```python
from build123d import *

# Parameters (mm, degrees)
SKETCH1_W           = 32.1
SKETCH1_H           = 32.1
SKETCH1_R           = 0.95
BOSS_EXTRUDE1_DEPTH = 1.65
SKETCH2_W           = 22.1
SKETCH2_H           = 6.75
BOSS_EXTRUDE2_DEPTH = 2.5
SKETCH3_R           = 0.625
BOSS_EXTRUDE3_DEPTH = 5
SKETCH4_R           = 7
BOSS_EXTRUDE4_DEPTH = 17


with BuildPart() as part:
    # Sketch1 → Boss-Extrude1 (new body)
    with BuildSketch(Plane(origin=(0, 0, 0), x_dir=(1, 0, 0), z_dir=(0, 1, 0))):
        Rectangle(SKETCH1_W, SKETCH1_H)
        with Locations(Location((-14.05, 14.05, 0), (0, 0, 270))):
            Circle(SKETCH1_R, mode=Mode.SUBTRACT)
        with Locations(Location((14.05, 14.05, 0), (0, 0, 90))):
            Circle(SKETCH1_R, mode=Mode.SUBTRACT)
        with Locations(Location((14.05, -14.05, 0), (0, 0, 270))):
            Circle(SKETCH1_R, mode=Mode.SUBTRACT)
        with Locations(Location((-14.05, -14.05, 0), (0, 0, 90))):
            Circle(SKETCH1_R, mode=Mode.SUBTRACT)
    extrude(amount=BOSS_EXTRUDE1_DEPTH)

    # Sketch2 → Boss-Extrude2 (add)
    with BuildSketch(Plane.XZ):
        with Locations((0, 12.675)):
            Rectangle(SKETCH2_W, SKETCH2_H)
    extrude(amount=BOSS_EXTRUDE2_DEPTH)

    # Sketch3 → Boss-Extrude3 (add)
    with BuildSketch(Plane(origin=(0, 1.65, 0), x_dir=(1, 0, 0), z_dir=(0, 1, 0))):
        with BuildLine():
            Line((9.9, 2.25), (8.55, 2.25))
            Line((8.55, 2.25), (8.55, 8.55))
            Line((8.55, 8.55), (-8.55, 8.55))
            Line((-8.55, 8.55), (-8.55, 2.25))
            Line((-8.55, 2.25), (-9.9, 2.25))
            ThreePointArc((-9.9, 2.25), (-12.15, 0), (-9.9, -2.25))
            Line((-9.9, -2.25), (-8.55, -2.25))
            Line((-8.55, -2.25), (-8.55, -8.55))
            Line((-8.55, -8.55), (8.55, -8.55))
            Line((8.55, -8.55), (8.55, -2.25))
            Line((8.55, -2.25), (9.9, -2.25))
            ThreePointArc((9.9, -2.25), (12.15, 0), (9.9, 2.25))
        make_face()
        with Locations(Location((9.9, 0, 0), (0, 0, 270))):
            Circle(SKETCH3_R, mode=Mode.SUBTRACT)
        with Locations(Location((-9.9, 0, 0), (0, 0, 90))):
            Circle(SKETCH3_R, mode=Mode.SUBTRACT)
    extrude(amount=BOSS_EXTRUDE3_DEPTH)

    # Sketch4 → Boss-Extrude4 (add)
    with BuildSketch(Plane(origin=(0, 6.65, 0), x_dir=(1, 0, 0), z_dir=(0, 1, 0))):
        with Locations(Location((0, 0, 0), (0, 0, 270))):
            Circle(SKETCH4_R)
    extrude(amount=BOSS_EXTRUDE4_DEPTH)


solid = part.part
```
The listing builds one solid part. Answer for the finished solid, in the listing's coordinates (mm). A direction names the side the tool comes from. Coordinates: 2 decimals unless noted, no trailing zeros. Write each loop counter-clockwise with the first axis right and the second up, starting at its lowest first coordinate (ties: lowest second). Pieces come first, ordered by that corner, then holes. Notation, with made-up numbers: M 7.25,9.5 L 61.25,9.5 A14 cw 61.25,20.5 Z; hole C -26,67.25 d7. An arc over 180 degrees is marked long. Use a Markdown table: item, result. Add a question column.
1. Section D-D (z = 10.5) is taken. Give the vertices of the cut face in (x, y).
2. Section C-C (x = 0) is taken. Give the vertices of the cut face in (y, z).
3. Which of the six approach directions +Z, -Z, +X, -X, +Y, -Y give full straight-line access (tool end or side, diameter ignored) to faces 1 (the flat face through (-9, 4, 2.25)), 2 (the flat face through (8.55, 4, -5)), 3 (the flat face through (10, 1.65, 0))?
4. Straight lines are drawn through the part: line 1 along X through (y, z) = (1.1, -14.05); line 2 along X through (y, z) = (3.85, 0) (3 decimals); line 3 along Y through (x, z) = (-12, -5.5). For each, find the intervals that lie inside material, in ascending order. Write a range as [from, to].
5. Given P1, Ø12, axis at x = 9.5, y = 20, coming from the +Z side; P2, Ø8, axis at x = -4.5, y = 10.5, coming from the +Z side; P3, Ø1.5, axis at y = 3.5, z = -4, coming from the +X side; P4, Ø3, axis at y = 14, z = -9.5, coming from the -X side, each flat-ended and moving along its own axis, determine where each tip first touches the part or whether it passes through.
6. Section B-B (y = 6) is taken. Give the vertices of the cut face in (x, z) (3 decimals).
7. Section A-A (z = -14.05) is taken. Give the vertices of the cut face in (x, y), plus the area to 3 significant figures.
8. For a pull along X with two mould halves and no side action, classify faces 4 (the cylindrical face through (-13.21, 0.81, 13.61)), 5 (the flat face through (11.05, -1, 13)), 6 (the flat face through (0, 4, -8.55)) as +X half, -X half, draft (parallel to the pull), parting line (faces both ways), or undercut.
Data:
| question | item | result |
|---|---|---|
| 1 | outline | M -16.05,0 L -11.05,0 L -11.05,-2.5 L 11.05,-2.5 L 11.05,0 L 16.05,0 L 16.05,1.65 L -16.05,1.65 Z |
| 2 | outline | M -2.5,9.3 L 0,9.3 L 0,-16.05 L 1.65,-16.05 L 1.65,-8.55 L 6.65,-8.55 L 6.65,-7 L 23.65,-7 L 23.65,7 L 6.65,7 L 6.65,8.55 L 1.65,8.55 L 1.65,16.05 L -2.5,16.05 Z |
| 3 | face 1 | +Z, -X, +Y |
| 3 | face 2 | -Z, +X, +Y |
| 3 | face 3 | +Y |
| 4 | line 1 | x = [-16.05, -15], [-13.1, 13.1], [15, 16.05] |
| 4 | line 2 | x = [-12.15, -10.525], [-9.275, 9.275], [10.525, 12.15] |
| 4 | line 3 | y = [0, 1.65] |
| 5 | P1 | stops at z = 6.06 |
| 5 | P2 | stops at z = 8.55 |
| 5 | P3 | stops at x = 8.55 |
| 5 | P4 | passes through |
| 6 | outline | M -9.9,-2.25 L -8.55,-2.25 L -8.55,-8.55 L 8.55,-8.55 L 8.55,-2.25 L 9.9,-2.25 A2.25 ccw 9.9,2.25 L 8.55,2.25 L 8.55,8.55 L -8.55,8.55 L -8.55,2.25 L -9.9,2.25 A2.25 ccw Z; hole C -9.9,0 d1.25; hole C 9.9,0 d1.25 |
| 7 | outline | M -16.05,0 L -15,0 L -15,1.65 L -16.05,1.65 Z; M -13.1,0 L 13.1,0 L 13.1,1.65 L -13.1,1.65 Z; M 15,0 L 16.05,0 L 16.05,1.65 L 15,1.65 Z |
| 7 | area | 46.7 mm2 |
| 8 | face 4 | undercut |
| 8 | face 5 | +X half |
| 8 | face 6 | draft |
